Verification items for this drawing (mm, ordinates from the low corner). Round coordinates to 2 decimals unless told otherwise and drop trailing zeros. Loops run counter-clockwise (first coordinate to the right, second up) from the corner with the lowest first, then second, coordinate; pieces in that order, holes last. Notation, with made-up numbers: (-27.5, 29) - (21.5, 29) arc R35 cw to (21.5, 68) - close; hole circle Ø9 at (82, 79). An arc over 180 degrees is marked (long way). Write item = value, one per line.
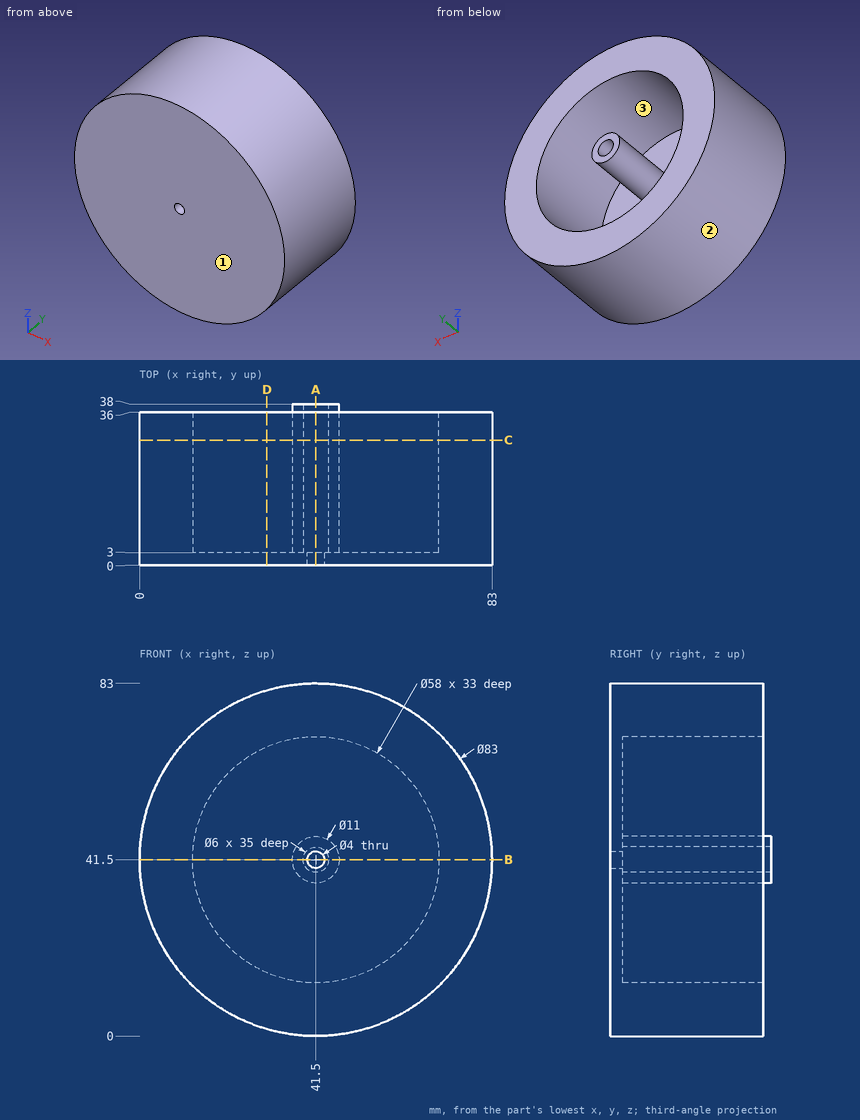
(1) Gauge pin test, flat ends, axial feed: pin 1 (3 mm diameter, centred on x = 51, z = 63, fed in from +Y); pin 2 (12 mm diameter, centred on x = 54, z = 17.5, fed in from +Y); pin 3 (4 mm diameter, centred on y = 15, z = 50, fed in from -X). Record the tip position at first contact, or that the pin passes through.
Answers follow:
pin_1 = 3
pin_2 = 36
pin_3 = 0.51
(2) Section check B-B (z = 41.5). Enter the section's corners in (x, y).
Answers follow:
outline = (0, 0) - (39.5, 0) - (39.5, 3) - (38.5, 3) - (38.5, 38) - (36, 38) - (36, 3) - (12.5, 3) - (12.5, 36) - (0, 36) - close; (43.5, 0) - (83, 0) - (83, 36) - (70.5, 36) - (70.5, 3) - (47, 3) - (47, 38) - (44.5, 38) - (44.5, 3) - (43.5, 3) - close
(3) Section check A-A (x = 41.5). Enter the section's corners in (y, z), then the cut area to 3 significant figures.
Answers follow:
outline = (0, 0) - (36, 0) - (36, 12.5) - (3, 12.5) - (3, 36) - (38, 36) - (38, 38.5) - (3, 38.5) - (3, 39.5) - (0, 39.5) - close; (0, 43.5) - (3, 43.5) - (3, 44.5) - (38, 44.5) - (38, 47) - (3, 47) - (3, 70.5) - (36, 70.5) - (36, 83) - (0, 83) - close
area = 1,240 mm²
(4) Section check D-D (x = 30). Enter the section's corners in (y, z).
Answers follow:
outline = (0, 1.63) - (36, 1.63) - (36, 14.88) - (3, 14.88) - (3, 68.12) - (36, 68.12) - (36, 81.37) - (0, 81.37) - close
(5) Scan lines: L1, parallel to Z at x = 41.5, y = 15; L2, parallel to Z at x = 44, y = 7.5. Record each from-to range of solid material in increasing order. Write a range as [from, to].
Answers follow:
L1 = [0, 12.5], [36, 38.5], [44.5, 47], [70.5, 83]
L2 = [0.08, 12.61], [36.6, 39.84], [43.16, 46.4], [70.39, 82.92]
(6) Section check C-C (y = 29.5). Enter the section's corners in (x, z), then the cut area to 3 significant figures.
Answers follow:
outline = circle Ø83 at (41.5, 41.5); circle Ø11 at (41.5, 41.5); hole circle Ø58 at (41.5, 41.5); hole circle Ø6 at (41.5, 41.5)
area = 2,840 mm²
(7) Mould release check, pull along Z, two halves, no side actions. Record for the marked faces 1, 2 and 3: pulls with the +Z half, pulls with the -Z half, needs draft (parallel to the pull), parting line crosses it, or undercut.
Answers follow:
face_1 = needs draft
face_2 = parting line crosses it
face_3 = undercut
